```python
from build123d import *

# Parameters (mm, degrees)
BOSS_EXTRUDE1_DEPTH = 5
TEETH_CUTOUT_DEPTH  = 6
FILLET2_R           = 0.5
SKETCH3_R           = 1.2
HOLE_CUTOUT_DEPTH   = 6
CUT_EXTRUDE1_DEPTH  = 6
FILLET3_R           = 1


with BuildPart() as part:
    # Sketch1 → Boss-Extrude1 (new body)
    with BuildSketch(Plane(origin=(0, 0, 0), x_dir=(1, 0, 0), z_dir=(0, 1, 0))):
        with BuildLine():
            Line((0, 0), (0, 30))
            Line((0, 30), (10, 47.320508076))
            Line((10, 47.320508076), (21.394885406, 80.413658222))
            Line((21.394885406, 80.413658222), (29.86, 85.73736322))
            ThreePointArc((29.86, 85.73736322), (34.475009673, 85.485348682), (35.771556302, 81.049044765))
            Line((35.771556302, 81.049044765), (24.157889764, 47.320508076))
            Line((24.157889764, 47.320508076), (21.394885406, 27.512282337))
            Line((21.394885406, 27.512282337), (27.71, 0))
            Line((27.71, 0), (0, 0))
        make_face()
    extrude(amount=BOSS_EXTRUDE1_DEPTH)

    # Sketch2 → Teeth_Cutout (cut, through all)
    with BuildSketch(Plane(origin=(0, 5, 0), x_dir=(1, 0, 0), z_dir=(0, 1, 0))):
        with BuildLine():
            ThreePointArc((35.771556302, 81.049044765), (31.958296112, 79.189193501), (33.818147375, 75.375933311))
            Line((33.818147375, 75.375933311), (35.771556302, 81.049044765))
        make_face()
        with BuildLine():
            ThreePointArc((32.841442912, 72.539377584), (29.028182721, 70.679526321), (30.888033985, 66.866266131))
            Line((30.888033985, 66.866266131), (32.841442912, 72.539377584))
        make_face()
        with BuildLine():
            ThreePointArc((29.911329522, 64.029710404), (26.098069331, 62.16985914), (27.957920595, 58.35659895))
            Line((27.957920595, 58.35659895), (29.911329522, 64.029710404))
        make_face()
        with BuildLine():
            ThreePointArc((26.981216131, 55.520043223), (23.167955941, 53.66019196), (25.027807205, 49.84693177))
            Line((25.027807205, 49.84693177), (26.981216131, 55.520043223))
        make_face()
        with BuildLine():
            ThreePointArc((24.111726827, 46.989561847), (20.726042313, 44.43277864), (23.28282552, 41.047094125))
            Line((23.28282552, 41.047094125), (24.111726827, 46.989561847))
        make_face()
        with BuildLine():
            Line((17.745535287, 30.930212077), (21.394885406, 27.512282337))
            Line((21.394885406, 27.512282337), (22.868374866, 38.075860265))
            Line((22.868374866, 38.075860265), (18.423003833, 35.787044768))
            ThreePointArc((18.423003833, 35.787044768), (16.82505927, 33.534272802), (17.745535287, 30.930212077))
        make_face()
        with BuildLine():
            Line((19.827305771, 16.086577823), (24.453138026, 14.188769628))
            Line((24.453138026, 14.188769628), (22.066045454, 24.588321976))
            Line((22.066045454, 24.588321976), (18.730897185, 20.863166138))
            ThreePointArc((18.730897185, 20.863166138), (18.042030328, 18.190917128), (19.827305771, 16.086577823))
        make_face()
        with BuildLine():
            Line((22.885558392, 2.763065114), (27.511390647, 0.865256919))
            Line((27.511390647, 0.865256919), (25.124298075, 11.264809267))
            Line((25.124298075, 11.264809267), (21.789149806, 7.539653429))
            ThreePointArc((21.789149806, 7.539653429), (21.100282948, 4.867404419), (22.885558392, 2.763065114))
        make_face()
    extrude(amount=-TEETH_CUTOUT_DEPTH, mode=Mode.SUBTRACT)

    # Fillet2
    fillet2_edges = [part.edges().sort_by_distance(p)[0] for p in [
        (27.71, 2.5, 0),
        (27.511390647, 2.5, -0.865256919),
    ]]
    fillet(fillet2_edges, radius=FILLET2_R)

    # Sketch3 → Hole_Cutout (cut, through all)
    with BuildSketch(Plane(origin=(0, 5, 0), x_dir=(1, 0, 0), z_dir=(0, 1, 0))):
        with Locations((11.72836197, 9.402231348)):
            Circle(SKETCH3_R)
        with Locations((9.432786312, 33.534272802)):
            Circle(SKETCH3_R)
        with Locations((17.675442081, 53.66019196)):
            Circle(SKETCH3_R)
        with Locations((27.173268391, 79.189193501)):
            Circle(SKETCH3_R)
    extrude(amount=-HOLE_CUTOUT_DEPTH, mode=Mode.SUBTRACT)

    # Sketch4 → Cut-Extrude1 (cut, through all)
    with BuildSketch(Plane(origin=(0, 5, 0), x_dir=(1, 0, 0), z_dir=(0, 1, 0))):
        Polygon((22.066045454, 24.588321976), (0, 24.588321976), (0, 0), (28.614713262, 0), (28.614713262, 24.588321976), align=None)
    extrude(amount=-CUT_EXTRUDE1_DEPTH, mode=Mode.SUBTRACT)

    # Fillet3
    fillet3_edges = [part.edges().sort_by_distance(p)[0] for p in [
        (0, 2.5, -24.588321976),
        (22.066045454, 2.5, -24.588321976),
    ]]
    fillet(fillet3_edges, radius=FILLET3_R)


solid = part.part
```
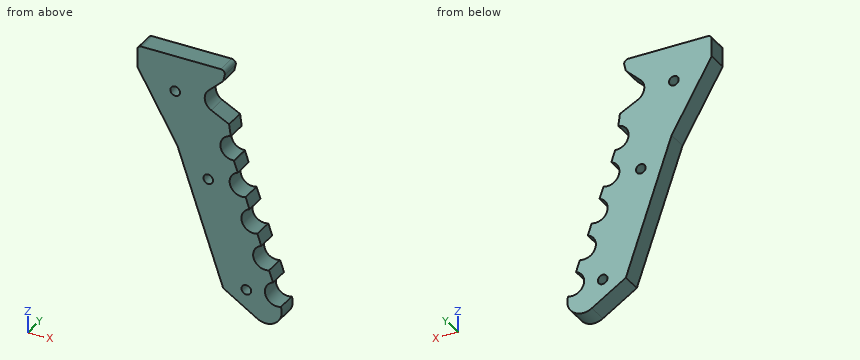
Model file for the job. Use its own axes, mm. Coordinates: 2 decimals unless noted, no trailing zeros. Write each loop counter-clockwise with the first axis right and the second up, starting at its lowest first coordinate (ties: lowest second). Pieces come first, ordered by that corner, then holes. Notation, with made-up numbers: (-5.5, 76) - (6.5, 76) arc R21 cw to (6.5, 110) - close; hole circle Ø11 at (23.25, -27.75). An arc over 180 degrees is marked (long way). One line per question, with ' | ' between items. Start each with the question number.
Q1. Cut at D-D, the plane x = 13. List the corners of the cut face in (y, z).
Q2. Cut at A-A, the plane y = 2.2. List the corners of the cut face in (x, z), then the cut area to 3 significant figures.
Q3. Cut at B-B, the plane x = 9. List the corners of the cut face in (y, z), then the cut area to 3 significant figures.
Q4. Drill centre lines: line 1 (X direction, y = 4.5, z = -33.5); line 2 (X direction, y = 2.8, z = -54); line 3 (Z direction, x = 9, y = 3.2). Where is each one in solid material? Low to high. Write a range as [from, to].
Q5. Pin check, flat tip, straight feed: pin 1 (1.5 mm diameter, centred on y = 2.5, z = -70.5, fed in from +X). Stop position of the tip, or through.
Q6. Cut at C-C, the plane z = -46. List the corners of the cut face in (x, y).
Answer below:
1) outline: (0, -56.03) - (5, -56.03) - (5, -24.59) - (0, -24.59) - close
2) outline: (0, -30) - (10, -47.32) - (21.39, -80.41) - (29.86, -85.74) arc R4 ccw to (35.77, -81.05) arc R3 cw to (33.82, -75.38) - (32.84, -72.54) arc R3 cw to (30.89, -66.87) - (29.91, -64.03) arc R3 cw to (27.96, -58.36) - (26.98, -55.52) arc R3 cw to (25.03, -49.85) - (24.16, -47.32) - (24.11, -46.99) arc R3 cw to (23.28, -41.05) - (22.87, -38.08) - (18.42, -35.79) arc R3 cw to (17.75, -30.93) - (21.39, -27.51) - (21.79, -25.81) arc R1 ccw to (20.81, -24.59) - (1, -24.59) arc R1 ccw to (0, -25.59) - close; hole circle Ø2.4 at (9.43, -33.53); hole circle Ø2.4 at (17.68, -53.66); hole circle Ø2.4 at (27.17, -79.19) | area: 830 mm^2
3) outline: (0, -45.59) - (5, -45.59) - (5, -34.65) - (0, -34.65) - close; (0, -32.42) - (5, -32.42) - (5, -24.59) - (0, -24.59) - close | area: 93.8 mm^2
4) line 1: [2.02, 8.23], [10.63, 16.82] | line 2: [12.3, 16.52], [18.83, 23.31] | line 3: [-45.59, -34.65], [-32.42, -24.59]
5) pin 1: x = 29.29
6) outline: (9.24, 0) - (21.44, 0) - (21.44, 5) - (9.24, 5) - close
